Geometry check sheet. Reference: drawing and pictorial views, mm from the part's lowest x, y, z. A direction names the side the tool comes from. Coordinates: 2 decimals unless noted, no trailing zeros. Loops run counter-clockwise (first coordinate to the right, second up) from the corner with the lowest first, then second, coordinate; pieces in that order, holes last. Notation, with made-up numbers: (-16.75, -25) -> (32.25, -25) arc R29 ccw to (32.25, 9) -> close; hole circle Ø8 at (45.25, -35.5). An arc over 180 degrees is marked (long way). Answer as a JSON object with one key per item and string values.
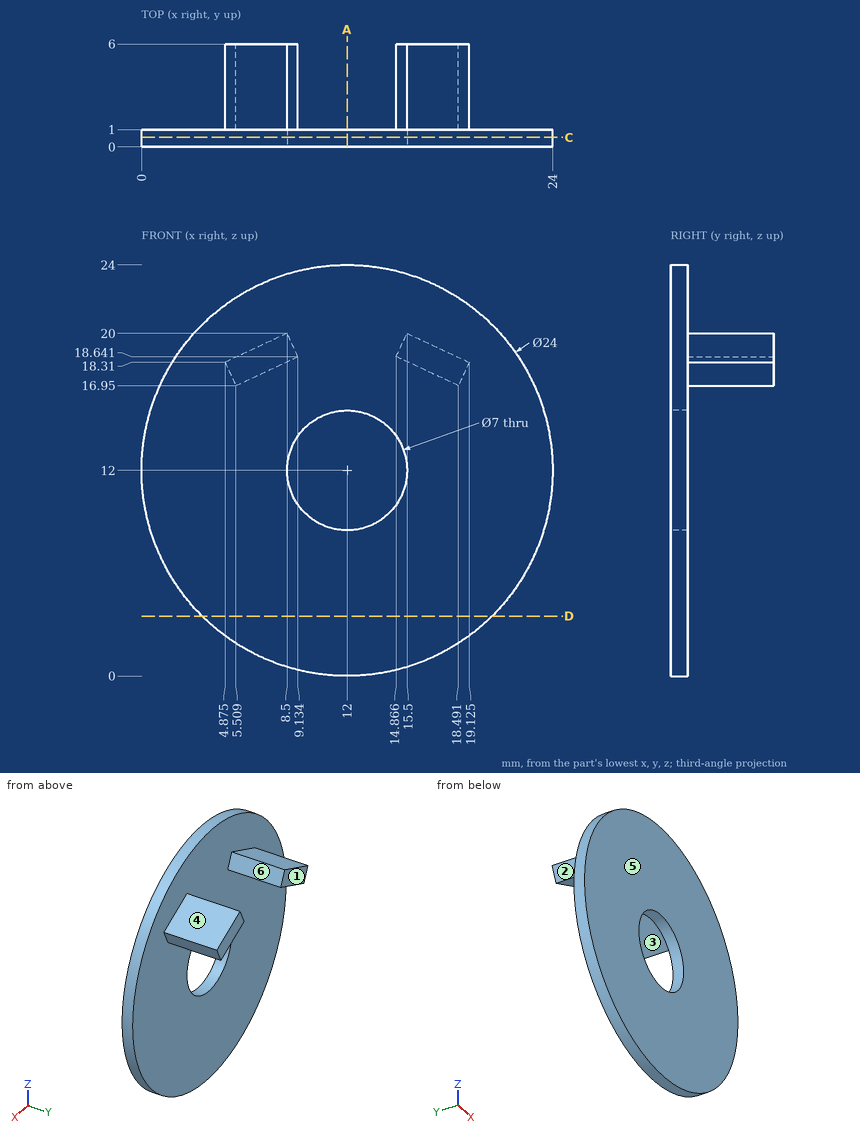
1. Section check D-D, the plane z = 3.5. Record the boundary of the cut face in (x, y).
Evaluation:
{"outline": "(3.53, 0) -> (20.47, 0) -> (20.47, 1) -> (3.53, 1) -> close"}
2. Tool access check on the marked faces 1, 2 and 3. Record the directions out of +Z, -Z, +X, -X, +Y, -Y that give a thin tool (end or side, any length) a straight path to the whole face; none if there is none.
Evaluation:
{"face 1": "+Z, -Z, +X, -X, +Y", "face 2": "-Z, -X, +Y", "face 3": "-Z, +Y"}
3. Section check A-A, the plane x = 12. Record the boundary of the cut face in (y, z).
Evaluation:
{"outline": "(0, 0) -> (1, 0) -> (1, 8.5) -> (0, 8.5) -> close; (0, 15.5) -> (1, 15.5) -> (1, 24) -> (0, 24) -> close"}
4. Mould release check, pull along X, two halves, no side actions. Record for the marked faces 4, 5 and 6: released by +X, released by -X, zero draft, split by the parting line, or undercut.
Evaluation:
{"face 4": "released by +X", "face 5": "zero draft", "face 6": "undercut"}
5. Depth check by flat-ended pin: P1, Ø2, axis at x = 18.5, z = 6, coming from the +Y side; P2, Ø3, axis at x = 8.5, y = 1.5, coming from the -Z side. Enter the tip coordinate at first touch or a pass-through.
Evaluation:
{"P1": "stops at y = 1", "P2": "stops at z = 0.18"}
6. Thickness scan on probe 1 along Z at (x, y) = (12, 0.35); probe 2 along Y at (x, z) = (5.5, 8.75). Record the ranges inside material, lowest first. Write a range as from..to.
Evaluation:
{"probe 1": "z = 0..8.5, 15.5..24", "probe 2": "y = 0..1"}
7. Section check C-C, the plane y = 0.55. Record the boundary of the cut face in (x, z).
Evaluation:
{"outline": "circle Ø24 at (12, 12); hole circle Ø7 at (12, 12)"}
